```python
from build123d import *

# Parameters (mm, degrees)
MAIN_PROFILE_DEPTH                              = 26
SKETCH2_W                                       = 18
SKETCH2_H                                       = 61.5
BODY_ATTACHMENT_CAVITY_DEPTH                    = 11.9
FILLET1_R                                       = 2.5
SKETCH5_W                                       = 24
SKETCH5_H                                       = 82
FACE_CAVITY_DEPTH                               = 4
FILLET2_R                                       = 2.5
CUT_EXTRUDE3_DEPTH                              = 4
FILLET3_R                                       = 2.5
SKETCH8_W                                       = 27.49705506
SKETCH8_H                                       = 110
CUT_REVOLVE1_ANGLE                              = 4
M3X0_5_TAPPED_HOLE1_D                           = 2.5
M3X0_5_TAPPED_HOLE1_DEPTH                       = 10
M3X0_5_TAPPED_HOLE1_TIP                         = 0.751075774
CSK_FOR_M4_FLAT_HEAD_MACHINE_SCREW1_D           = 4.5
CSK_FOR_M4_FLAT_HEAD_MACHINE_SCREW1_DEPTH       = 10
CSK_FOR_M4_FLAT_HEAD_MACHINE_SCREW1_CSINK_D     = 9.4
CSK_FOR_M4_FLAT_HEAD_MACHINE_SCREW1_CSINK_ANGLE = 90
CSK_FOR_M4_FLAT_HEAD_MACHINE_SCREW1_TIP         = 1.351936393
F_3_32_0_09375_DIAMETER_HOLE1_D                 = 2.38125
F_3_32_0_09375_DIAMETER_HOLE1_DEPTH             = 5.284600325
F_3_32_0_09375_DIAMETER_HOLE1_TIP               = 0.715399675
FILLET4_R                                       = 1


with BuildPart() as part:
    # Sketch1 → Main Profile (new body)
    with BuildSketch(Plane.XY):
        Polygon((-2.5, 55), (-12.5, 43), (-12.5, -43), (-2.5, -55), (0.5, -55), (12.5, 0), (0.5, 55), align=None)
    extrude(amount=MAIN_PROFILE_DEPTH)

    # Sketch2 → Body Attachment Cavity (cut)
    with BuildSketch(Plane.ZY.offset(-12.5)):
        with Locations((9, 0)):
            Rectangle(SKETCH2_W, SKETCH2_H)
    extrude(amount=BODY_ATTACHMENT_CAVITY_DEPTH, mode=Mode.SUBTRACT)

    # Fillet1
    fillet1_edges = [part.edges().sort_by_distance(p)[0] for p in [
        (0.6, -30.75, 9),
        (0.6, 30.75, 9),
    ]]
    fillet(fillet1_edges, radius=FILLET1_R)

    # Sketch5 → Face Cavity (cut)
    with BuildSketch(Plane.ZY.offset(12.5)):
        with Locations((12, 0)):
            Rectangle(SKETCH5_W, SKETCH5_H)
    extrude(amount=-FACE_CAVITY_DEPTH, mode=Mode.SUBTRACT)

    # Fillet2
    fillet2_edges = [part.edges().sort_by_distance(p)[0] for p in [
        (-10.5, 41, 24),
        (-10.5, -41, 24),
    ]]
    fillet(fillet2_edges, radius=FILLET2_R)

    # Sketch7 → Cut-Extrude3 (cut)
    with BuildSketch(Plane(origin=(0, 0, 0), x_dir=(-1, 0, 0), z_dir=(0, 0, -1))):
        Polygon((10.5, 41), (1.077337627, 52.021045042), (1.077337627, -52.021045042), (10.5, -41), align=None)
    extrude(amount=-CUT_EXTRUDE3_DEPTH, mode=Mode.SUBTRACT)

    # Fillet3
    fillet3_edges = [part.edges().sort_by_distance(p)[0] for p in [
        (-1.077337627, -52.021045042, 2),
        (-1.077337627, 52.021045042, 2),
    ]]
    fillet(fillet3_edges, radius=FILLET3_R)

    # Sketch8 → Cut-Revolve1 (revolve, cut)
    with BuildSketch(Plane.ZY.offset(12.5)):
        with Locations((13.74852753, -6)):
            Rectangle(SKETCH8_W, SKETCH8_H)
    revolve(axis=Axis((-12.5, 49, 0), (0, 1, 0)), revolution_arc=CUT_REVOLVE1_ANGLE, mode=Mode.SUBTRACT)

    # M3x0.5 Tapped Hole1
    with Locations(Plane(origin=(0, 0, 4), x_dir=(-1, 0, 0), z_dir=(0, 0, -1))):
        with Locations((5.25, 40.95), (5.25, -40.95)):
            Hole(M3X0_5_TAPPED_HOLE1_D / 2, depth=M3X0_5_TAPPED_HOLE1_DEPTH)
            with Locations((0, 0, -(M3X0_5_TAPPED_HOLE1_DEPTH + M3X0_5_TAPPED_HOLE1_TIP / 2))):  # 118° drill point
                Cone(0, M3X0_5_TAPPED_HOLE1_D / 2, M3X0_5_TAPPED_HOLE1_TIP, mode=Mode.SUBTRACT)

    # CSK for M4 Flat Head Machine Screw1
    with Locations(Plane.ZY.offset(8.5)):
        with Locations((10.5, 20.5), (10.5, -20.5)):
            CounterSinkHole(CSK_FOR_M4_FLAT_HEAD_MACHINE_SCREW1_D / 2, CSK_FOR_M4_FLAT_HEAD_MACHINE_SCREW1_CSINK_D / 2, depth=CSK_FOR_M4_FLAT_HEAD_MACHINE_SCREW1_DEPTH, counter_sink_angle=CSK_FOR_M4_FLAT_HEAD_MACHINE_SCREW1_CSINK_ANGLE)
            with Locations((0, 0, -(CSK_FOR_M4_FLAT_HEAD_MACHINE_SCREW1_DEPTH + CSK_FOR_M4_FLAT_HEAD_MACHINE_SCREW1_TIP / 2))):  # 118° drill point
                Cone(0, CSK_FOR_M4_FLAT_HEAD_MACHINE_SCREW1_D / 2, CSK_FOR_M4_FLAT_HEAD_MACHINE_SCREW1_TIP, mode=Mode.SUBTRACT)

    # 3/32 (0.09375) Diameter Hole1
    with Locations(Plane(origin=(0, 0, 18), x_dir=(-1, 0, 0), z_dir=(0, 0, -1))):
        with Locations((-3.193818752, 28.18337425), (-3.193818752, -28.18337425)):
            Hole(F_3_32_0_09375_DIAMETER_HOLE1_D / 2, depth=F_3_32_0_09375_DIAMETER_HOLE1_DEPTH)
            with Locations((0, 0, -(F_3_32_0_09375_DIAMETER_HOLE1_DEPTH + F_3_32_0_09375_DIAMETER_HOLE1_TIP / 2))):  # 118° drill point
                Cone(0, F_3_32_0_09375_DIAMETER_HOLE1_D / 2, F_3_32_0_09375_DIAMETER_HOLE1_TIP, mode=Mode.SUBTRACT)

    # Fillet4
    fillet4_edges = [part.edges().sort_by_distance(p)[0] for p in [
        (-6.590951445, -50.090858266, 26),
        (-6.590951445, 50.090858266, 26),
        (-10.681902889, 0, 26),
        (-2.5, 55, 13),
        (0.5, 55, 13),
        (0.5, -55, 13),
        (-2.5, -55, 13),
        (-1, -55, 26),
        (6.5, -27.5, 26),
        (6.5, 27.5, 26),
        (-1, 55, 26),
    ]]
    fillet(fillet4_edges, radius=FILLET4_R)


solid = part.part
```
Geometry check sheet. Reference: the model listing, model coordinates, mm. A direction names the side the tool comes from. Give positions to 0.01 mm unless a question says otherwise; leave off trailing zeros. Write each loop counter-clockwise with the first axis right and the second up, starting at its lowest first coordinate (ties: lowest second). Pieces come first, ordered by that corner, then holes.
1) Gauge pin test, flat ends, axial feed: pin 1 (9 mm diameter, centred on y = -8, z = 7.5, fed in from +X); pin 2 (1.9 mm diameter, centred on x = -9, y = 4.5, fed in from -Z); pin 3 (6 mm diameter, centred on y = -20.5, z = 10.5, fed in from -X). Record the tip position at first contact, or that the pin passes through.
2) Release check for a two-part mould opening along Y. For faces 1 (the cylindrical face through (-6.61, 49.62, 25.7)), 2 (the cylindrical face through (6.39, -26.67, 25.7)), 3 (the flat face through (0.6, 0, 9)) record: pulls with the +Y half, pulls with the -Y half, needs draft (parallel to the pull), parting line crosses it, or undercut.
3) Material ranges on L1, parallel to Y at x = -2, z = 10.5; L2, parallel to Y at x = -5.25, z = 9; L3, parallel to Z at x = -3.75, y = -20.5, recorded low to high.
4) Access from +Z, -Z, +X, -X, +Y, -Y to the whole of each face (thin tool, end or side, straight path). Record for faces 4 (the flat face through (5, 0, 18)), 5 (the cylindrical face through (-9.731, -40.287, 23.248)), 6 (the cylindrical face through (3.74, -29.24, 20.68)), 7 (the flat face through (-10.784, -3.13, 24.547)).
5) Section check A-A, the plane z = 10.5. State how many separate pieces and enclosed holes the cut face has, and give its area (3 significant figures).
6) Section check B-B, the plane z = 1.5. Record the boundary of the cut face in (x, y), and give its area (3 significant figures).
7) Section check C-C, the plane z = 20.25. Record the boundary of the cut face in (x, y).
Computed:
1. pin 1: stops at x = 0.6
1. pin 2: stops at z = 4
1. pin 3: stops at x = -6.8
2. face 1: pulls with the +Y half
2. face 2: pulls with the -Y half
2. face 3: undercut
3. L1: y = -55 to -22.75, -18.25 to 18.25, 22.75 to 55
3. L2: y = -51.7 to -42.2, -39.7 to -22.18, -18.82 to 18.82, 22.18 to 39.7, 42.2 to 51.7
3. L3: z = 4 to 8.25, 12.75 to 26
4. face 4: -Z, +X
4. face 5: -Z, -X
4. face 6: -Z
4. face 7: +Z, -X, +Y, -Y
5. separate pieces: 3
5. enclosed holes: 2
5. area: 1,010 mm2
6. outline: (-12.4, -43.13) - (-2.8, -54.64) arc R1 ccw to (-2.03, -55) - (-0.31, -55) arc R1 ccw to (0.67, -54.21) - (5.79, -30.75) - (3.1, -30.75) arc R2.5 cw to (0.6, -28.25) - (0.6, 28.25) arc R2.5 cw to (3.1, 30.75) - (5.79, 30.75) - (0.67, 54.21) arc R1 ccw to (-0.31, 55) - (-2.03, 55) arc R1 ccw to (-2.8, 54.64) - (-12.4, 43.13) - (-12.4, 41) - (-10.5, 41) - (-5.48, 46.87) arc R2.5 cw to (-1.08, 45.25) - (-1.08, -45.25) arc R2.5 cw to (-5.48, -46.87) - (-10.5, -41) - (-12.4, -41) - close
6. area: 425 mm2
7. outline: (-11.08, -44.7) - (-2.8, -54.64) arc R1 ccw to (-2.03, -55) - (-0.31, -55) arc R1 ccw to (0.67, -54.21) - (12.5, 0) - (0.67, 54.21) arc R1 ccw to (-0.31, 55) - (-2.03, 55) arc R1 ccw to (-2.8, 54.64) - (-11.08, 44.7) - (-11.08, 41) - (-8.5, 41) - (-8.5, -41) - (-11.08, -41) - close; hole circle Ø2.38 at (3.19, -28.18); hole circle Ø2.38 at (3.19, 28.18)
